```python
from build123d import *

# Parameters (mm, degrees)
SHELL_1_T = -3


with BuildPart() as part:
    # 草图1 → 旋转1 (revolve)
    with BuildSketch(Plane.XY, mode=Mode.PRIVATE) as revolve_1_sk:
        Polygon((0, 0), (-90, 0), (-105, 185), (-120, 185), (-120, 200), (0, 200), align=None)
    revolve(revolve_1_sk.sketch.rotate(Axis((0, -878.981608445, 0), (0, 1, 0)), 180), axis=Axis((0, -878.981608445, 0), (0, 1, 0)))

    # 抽壳1
    shell_1_openings = [part.faces().sort_by_distance(p)[0] for p in [
        (0, 200, 0),
    ]]
    offset(amount=SHELL_1_T, openings=shell_1_openings, kind=Kind.INTERSECTION)


solid = part.part
```
Design review of the part built by this model. Coordinates are the model's own, in mm. A direction names the side the tool comes from. Coordinates: 2 decimals unless noted, no trailing zeros. Write each loop counter-clockwise with the first axis right and the second up, starting at its lowest first coordinate (ties: lowest second). Pieces come first, ordered by that corner, then holes. Notation, with made-up numbers: M 45.25,-38 L 55.25,-38 A27 cw 55.25,-7 Z; hole C -31.5,2.5 d11. An arc over 180 degrees is marked long. Answer as a JSON object with one key per item and string values.
Item 1: Machinability: for faces 5 (the cylindrical face through (64.511, 192.605, -101.184)), 6 (the flat face through (1, 188, 103)), 7 (the flat face through (1, 185, 106)), which of the approach directions +Z, -Z, +X, -X, +Y, -Y give a long, thin tool a straight path to every point of the face, cutting with its end or side? Answer none if there is none.
Outcome:
{"face 5": "+Y, -Y", "face 6": "+Y", "face 7": "-Y"}
Item 2: Add section B-B, the plane z = 0. Give the boundary of the cut face in (x, y), and give its area (3 significant figures).
Outcome:
{"outline": "M -120,185 L -105,185 L -90,0 L 90,0 L 105,185 L 120,185 L 120,200 L 117,200 L 117,188 L 102.23,188 L 87.23,3 L -87.23,3 L -102.23,188 L -117,188 L -117,200 L -120,200 Z", "area": "1,820 mm²"}
Item 3: Add section C-C, the plane y = 27.5. Give the boundary of the cut face in (x, z), and give its area (3 significant figures).
Outcome:
{"outline": "C 0,0 d184.46; hole C 0,0 d178.44", "area": "1,720 mm²"}
Item 4: Wall thickness on probe 1 along X at (y, z) = (191.5, 1); probe 2 along Y at (x, z) = (83.5, -81.5): over which ranges is each line inside the solid? List them lowest first.
Outcome:
{"probe 1": "-120 to -117, 117 to 120", "probe 2": "185 to 188"}
Item 5: Insertion check: pin 1 Ø10 at (x, y) = (-56, 179.5) entering from -Z; pin 2 Ø12 at (x, z) = (22, -84.5) entering from -Y; pin 3 Ø3 at (y, z) = (44, -57) entering from +X; pin 4 Ø10 at (y, z) = (97, 93.5) entering from -X. Each pin has a flat end and moves straight along its axis. Give the tip position at first contact, or say it passes through.
Outcome:
{"pin 1": "z = -91.31", "pin 2": "y = 0", "pin 3": "x = 75.34", "pin 4": "x = -41.82"}
Item 6: Add section A-A, the plane x = 0. Give the boundary of the cut face in (y, z), and give its area (3 significant figures).
Outcome:
{"outline": "M 0,-90 L 185,-105 L 185,-120 L 200,-120 L 200,-117 L 188,-117 L 188,-102.23 L 3,-87.23 L 3,87.23 L 188,102.23 L 188,117 L 200,117 L 200,120 L 185,120 L 185,105 L 0,90 Z", "area": "1,820 mm²"}
Item 7: Draft analysis for pull direction Z (two halves, no side actions). For faces 1 (the conical face through (93.098, 93.795, -29.318)), 2 (the flat face through (1, 3, -1)), 3 (the flat face through (26, 200, 115)), 4 (the cylindrical face through (111.6, 194.08, -35.14)), state which applies: pulls with the +Z half, pulls with the -Z half, needs draft (parallel to the pull), parting line crosses it, or undercut.
Outcome:
{"face 1": "parting line crosses it", "face 2": "undercut", "face 3": "needs draft", "face 4": "undercut"}
Item 8: Add section D-D, the plane y = 162.5. Give the boundary of the cut face in (x, z).
Outcome:
{"outline": "C 0,0 d206.35; hole C 0,0 d200.33"}
